Input: part model. Units: mm. Frame: model coordinates. Face numbers are marked on the shaded views. A direction names the side the tool comes from. Give positions to 0.01 mm unless a question says otherwise; leave off trailing zeros. Write each loop counter-clockwise with the first axis right and the second up, starting at its lowest first coordinate (ties: lowest second). Pieces come first, ordered by that corner, then holes. Notation, with made-up numbers: (-39.75, 1) - (-17.75, 1) arc R12 cw to (-17.75, 8) - close; hole circle Ø6 at (18.25, -29.75). An arc over 180 degrees is marked (long way). Answer as a JSON object with one key per item and string values. Group by question number.
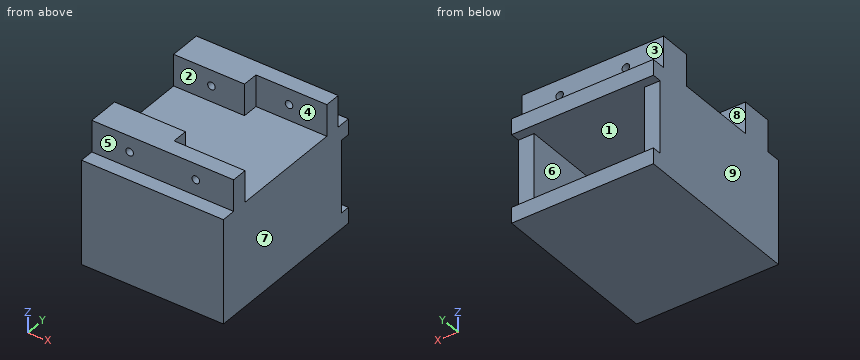
from build123d import *

# Parameters (mm, degrees)
SKETCH_1_W          = 45
SKETCH_1_H          = 50
EXTRUDE_1_DEPTH     = 43
SKETCH_2_W          = 35
SKETCH_2_H          = 23
CUT_EXTRUDE_1_DEPTH = 70.679623994
SKETCH_3_W          = 45
SKETCH_3_H          = 43
EXTRUDE_2_DEPTH     = 5
SKETCH_4_W          = 10
SKETCH_4_H          = 26
SKETCH_4_H_2        = 4.5
CUT_EXTRUDE_2_DEPTH = 70.09413868
SKETCH_5_W          = 22.5
SKETCH_5_H          = 5
CUT_EXTRUDE_3_DEPTH = 10
HOLE_WIZARD_M2_1_D  = 2.4
SKETCH_8_W          = 45
SKETCH_8_H          = 23
CUT_EXTRUDE_4_DEPTH = 3
CUT_EXTRUDE_5_REACH = 59.055
SKETCH_11_W         = 22.5
SKETCH_11_H         = 5


with BuildPart() as part:
    # ｽｹｯﾁ1 → ﾎﾞｽ - 押し出し1 (new body)
    with BuildSketch(Plane.XY):
        Rectangle(SKETCH_1_W, SKETCH_1_H)
    extrude(amount=EXTRUDE_1_DEPTH)

    # ｽｹｯﾁ2 → ｶｯﾄ - 押し出し1 (cut, through all)
    with BuildSketch(Plane(origin=(0, 25, 0), x_dir=(1, 0, 0), z_dir=(0, 1, 0))):
        with Locations((0, -16.5)):
            Rectangle(SKETCH_2_W, SKETCH_2_H)
    extrude(amount=-CUT_EXTRUDE_1_DEPTH, mode=Mode.SUBTRACT)

    # ｽｹｯﾁ3 → ﾎﾞｽ - 押し出し2 (add)
    with BuildSketch(Plane.XZ.offset(25)):
        with Locations((0, 21.5)):
            Rectangle(SKETCH_3_W, SKETCH_3_H)
    extrude(amount=EXTRUDE_2_DEPTH)

    # ｽｹｯﾁ4 → ｶｯﾄ - 押し出し2 (cut, through all)
    with BuildSketch(Plane(origin=(22.5, 0, 0), x_dir=(0, 0, -1), z_dir=(1, 0, 0))):
        with Locations((-38, -2.5)):
            Rectangle(SKETCH_4_W, SKETCH_4_H)
        with Locations((-38, -27.75)):
            Rectangle(SKETCH_4_W, SKETCH_4_H_2)
        with Locations((-38, 22.75)):
            Rectangle(SKETCH_4_W, SKETCH_4_H_2)
    extrude(amount=-CUT_EXTRUDE_2_DEPTH, mode=Mode.SUBTRACT)

    # ｽｹｯﾁ5 → ｶｯﾄ - 押し出し3 (cut)
    with BuildSketch(Plane.XY.offset(43)):
        with Locations((11.25, 13)):
            Rectangle(SKETCH_5_W, SKETCH_5_H)
    extrude(amount=-CUT_EXTRUDE_3_DEPTH, mode=Mode.SUBTRACT)

    # M2 すきま穴1 (through all)
    with Locations(Plane(origin=(0, 20.5, 0), x_dir=(1, 0, 0), z_dir=(0, 1, 0))):
        with Locations((-10.5, -38), (10.5, -38)):
            Hole(HOLE_WIZARD_M2_1_D / 2)

    # ｽｹｯﾁ8 → ｶｯﾄ - 押し出し4 (cut)
    with BuildSketch(Plane(origin=(0, 25, 0), x_dir=(1, 0, 0), z_dir=(0, 1, 0))):
        with Locations((0, -16.5)):
            Rectangle(SKETCH_8_W, SKETCH_8_H)
    extrude(amount=-CUT_EXTRUDE_4_DEPTH, mode=Mode.SUBTRACT)

    # ｶｯﾄ - 押し出し5: up to this face of the body (flat: up to its plane)
    cut_extrude_5_end = Plane(part.part.faces().sort_by_distance((0.986842105, -1.140350877, 33))[0])
    # ｽｹｯﾁ11 → ｶｯﾄ - 押し出し5 (cut, up to the picked face)
    with BuildSketch(Plane.XY.offset(43), mode=Mode.PRIVATE) as cut_extrude_5_sk1:
        with Locations((11.25, -18)):
            Rectangle(SKETCH_11_W, SKETCH_11_H)
    cut_extrude_5_tool1 = split(extrude(cut_extrude_5_sk1.sketch, amount=-CUT_EXTRUDE_5_REACH, mode=Mode.PRIVATE), bisect_by=cut_extrude_5_end, keep=Keep.BOTH, mode=Mode.PRIVATE)
    add(cut_extrude_5_tool1.solids().sort_by(Axis((11.25, -18, 43), (0, 0, -1)))[0], mode=Mode.SUBTRACT)


solid = part.part
1) Cut plane C-C on y = -6. Return the cut outline in (x, z), and give its area (3 significant figures).
2) Cut plane B-B on z = 38. Return the cut outline in (x, y).
3) Reachability of the marked faces 1, 2, 3, 4 and 5 from +Z, -Z, +X, -X, +Y, -Y: full face, straight path, thin tool, end or side. Return the list, or none.
4) Cut plane A-A on x = 10.5. Return the cut outline in (y, z), and give its area (3 significant figures).
5) Mould query, pull axis X, two halves, no side actions, for the marked faces 6, 7, 8 and 9. Classes: +X half, -X half, draft (parallel to the pull), parting line (faces both ways), or undercut.
6) Line query: line 1 along X through (y, z) = (17.5, 38); line 2 along Z through (x, y) = (10.5, 18.1); line 3 along Z through (x, y) = (15.5, -7). Output: solid intervals per line, ascending. Write a range as from..to.
7) Cut plane D-D on y = -16.5. Return the cut outline in (x, z), and give its area (3 significant figures).
8) Pin query (flat end, axial travel): P1, Ø6, axis at x = 3, y = 18, coming from the -Z side; P2, Ø6, axis at x = -5.5, y = 3, coming from the +Z side; P3, Ø5, axis at y = -14, z = 37, coming from the +X side; P4, Ø3, axis at x = 10.5, z = 40, coming from the -Y side. Return the tip coordinate at first contact, or that it passes through.
Filled in:
{
 "1": {"outline": "(-22.5, 0) - (22.5, 0) - (22.5, 33) - (-22.5, 33) - close; hole (-17.5, 5) - (17.5, 5) - (17.5, 28) - (-17.5, 28) - close", "area": "680 mm²"},
 "2": {"outline": "(-22.5, -25.5) - (-11.7, -25.5) - (-11.7, -15.5) - (-22.5, -15.5) - close; (-22.5, 10.5) - (-11.7, 10.5) - (-11.7, 20.5) - (-22.5, 20.5) - close; (-9.3, -25.5) - (9.3, -25.5) - (9.3, -20.5) - (0, -20.5) - (0, -15.5) - (-9.3, -15.5) - close; (-9.3, 10.5) - (0, 10.5) - (0, 15.5) - (9.3, 15.5) - (9.3, 20.5) - (-9.3, 20.5) - close; (11.7, -25.5) - (22.5, -25.5) - (22.5, -20.5) - (11.7, -20.5) - close; (11.7, 15.5) - (22.5, 15.5) - (22.5, 20.5) - (11.7, 20.5) - close"},
 "3": {"face 1": "+Y", "face 2": "+Z, +X, -X", "face 3": "+Z, +X, -X, +Y", "face 4": "+Z, +X", "face 5": "+Z, +X, -X, -Y"},
 "4": {"outline": "(-30, 0) - (25, 0) - (25, 5) - (-25, 5) - (-25, 28) - (25, 28) - (25, 33) - (20.5, 33) - (20.5, 36.8) - (15.5, 36.8) - (15.5, 33) - (-20.5, 33) - (-20.5, 36.8) - (-25.5, 36.8) - (-25.5, 33) - (-30, 33) - close; (-25.5, 39.2) - (-20.5, 39.2) - (-20.5, 43) - (-25.5, 43) - close; (15.5, 39.2) - (20.5, 39.2) - (20.5, 43) - (15.5, 43) - close", "area": "741 mm²"},
 "5": {"face 6": "undercut", "face 7": "+X half", "face 8": "draft", "face 9": "-X half"},
 "6": {"line 1": "x = -22.5..-11.7, -9.3..9.3, 11.7..22.5", "line 2": "z = 0..5, 28..36.8, 39.2..43", "line 3": "z = 0..5, 28..33"},
 "7": {"outline": "(-22.5, 0) - (22.5, 0) - (22.5, 33) - (0, 33) - (0, 43) - (-22.5, 43) - close; hole (-17.5, 5) - (17.5, 5) - (17.5, 28) - (-17.5, 28) - close; hole circle Ø2.4 at (-10.5, 38)", "area": "900 mm²"},
 "8": {"P1": "stops at z = 0", "P2": "stops at z = 33", "P3": "stops at x = 0", "P4": "stops at y = -25.5"}
}
